Source: CAD feature listing. Evaluate the final solid. Frame: model axes, mm. A direction names the side the tool comes from. Give positions to 0.01 mm unless a question says otherwise; leave off trailing zeros. Loops run counter-clockwise (first coordinate to the right, second up) from the corner with the lowest first, then second, coordinate; pieces in that order, holes last. Notation, with made-up numbers: M 79.25,-28.75 L 101.25,-28.75 A21 ccw 101.25,10.25 Z; hole C 68.25,2.5 d7. An arc over 180 degrees is marked long. Write item = value, one per line.
from build123d import *

# Parameters (mm, degrees)
F0_W      = 315
F0_H      = 155
F1_DEPTH  = 105
F2_W      = 118
F2_H      = 80
F3_DEPTH  = 70
F4_W      = 65
F4_H      = 50
F5_DEPTH  = 57
F6_W      = 150
F6_H      = 15
F7_DEPTH  = 100
F8_W      = 150
F8_H      = 12
F9_DEPTH  = 75
F10_W     = 55
F10_H     = 28
F11_DEPTH = 55
F12_W     = 70
F12_H     = 30
F13_DEPTH = 100
F14_W     = 90
F14_H     = 20
F15_DEPTH = 90


with BuildPart() as f1:
    # F0 (on Top) → F1 (new body)
    with BuildSketch(Plane.XY):
        with Locations((-126.290321, 61.441531)):
            Rectangle(F0_W, F0_H)
    extrude(amount=F1_DEPTH)

    # F2 (on face) → F3 (cut)
    with BuildSketch(Plane.XY.offset(105)):
        with Locations((-41.790321, 37.941531)):
            Rectangle(F2_W, F2_H)
    extrude(amount=-F3_DEPTH, mode=Mode.SUBTRACT)

    # F4 (on face) → F5 (cut)
    with BuildSketch(Plane.XY.offset(105)):
        with Locations((-237.290321, 80.884401)):
            Rectangle(F4_W, F4_H)
    extrude(amount=-F5_DEPTH, mode=Mode.SUBTRACT)

    # F6 (on face) → F7 (cut)
    with BuildSketch(Plane.XY.offset(105)):
        with Locations((-194.790321, 5.441531)):
            Rectangle(F6_W, F6_H)
    extrude(amount=-F7_DEPTH, mode=Mode.SUBTRACT)

    # F8 (on face) → F9 (cut)
    with BuildSketch(Plane.XY.offset(105)):
        with Locations((-194.790321, 32.941531)):
            Rectangle(F8_W, F8_H)
    extrude(amount=-F9_DEPTH, mode=Mode.SUBTRACT)

    # F10 (on face) → F11 (cut)
    with BuildSketch(Plane.XY.offset(105)):
        with Locations((-147.290321, 66.941531)):
            Rectangle(F10_W, F10_H)
    extrude(amount=-F11_DEPTH, mode=Mode.SUBTRACT)

    # F12 (on face) → F13 (cut)
    with BuildSketch(Plane.XY.offset(105)):
        with Locations((-154.790321, 109.941531)):
            Rectangle(F12_W, F12_H)
    extrude(amount=-F13_DEPTH, mode=Mode.SUBTRACT)

    # F14 (on face) → F15 (cut)
    with BuildSketch(Plane.XY.offset(105)):
        with Locations((-55.790321, 104.941531)):
            Rectangle(F14_W, F14_H)
    extrude(amount=-F15_DEPTH, mode=Mode.SUBTRACT)


solid = f1.part
1. Cut plane C-C, the plane y = 99. Return the cut outline in (x, z).
Derived:
outline = M -283.79,0 L 31.21,0 L 31.21,105 L -10.79,105 L -10.79,15 L -100.79,15 L -100.79,105 L -119.79,105 L -119.79,5 L -189.79,5 L -189.79,105 L -204.79,105 L -204.79,48 L -269.79,48 L -269.79,105 L -283.79,105 Z
2. Cut plane A-A, the plane z = 22.5. Return the cut outline in (x, y), then the cut area to 3 significant figures.
Derived:
outline = M -283.79,-16.06 L 31.21,-16.06 L 31.21,138.94 L -283.79,138.94 Z; hole M -269.79,-2.06 L -119.79,-2.06 L -119.79,12.94 L -269.79,12.94 Z; hole M -189.79,94.94 L -119.79,94.94 L -119.79,124.94 L -189.79,124.94 Z; hole M -100.79,94.94 L -10.79,94.94 L -10.79,114.94 L -100.79,114.94 Z
area = 42,700 mm²
3. Material intervals for probe 1 along X at (y, z) = (35, 63.5); probe 2 along Y at (x, z) = (-44.5, 92); probe 3 along Y at (x, z) = (-202.5, 87), sorted ascending. Write a range as from..to.
Derived:
probe_1 = -283.79..-269.79, -119.79..-100.79, 17.21..31.21
probe_2 = -16.06..-2.06, 77.94..94.94, 114.94..138.94
probe_3 = -16.06..-2.06, 12.94..26.94, 38.94..138.94
4. Pull-direction query (Y, two-part tool) for faces 3 (the flat face through (-128, 138.942, 52)), 4 (the flat face through (-128, 45, 105)), 5 (the flat face through (-155, 110, 5)); classes: +Y half, -Y half, draft (parallel to the pull), parting line (faces both ways), or undercut.
Derived:
face_3 = +Y half
face_4 = draft
face_5 = undercut
5. Reachability of faces 1 (the flat face through (-196, 26.942, 68)), 2 (the flat face through (-283.79, 60, 52)) from +Z, -Z, +X, -X, +Y, -Y: full face, straight path, thin tool, end or side. Return the list, or none.
Derived:
face_1 = +Z
face_2 = +Z, -Z, -X, +Y, -Y
6. Cut plane D-D, the plane z = 68.5. Count the separate pieces of the cut face and the enclosed holes in it, then the cut area to 3 significant figures.
Derived:
separate_pieces = 1
enclosed_holes = 7
area = 26,600 mm²
7. Cut plane B-B, the plane x = -152. Return the cut outline in (y, z), then the cut area to 4 significant figures.
Derived:
outline = M -16.06,0 L 138.94,0 L 138.94,105 L 124.94,105 L 124.94,5 L 94.94,5 L 94.94,105 L 80.94,105 L 80.94,50 L 52.94,50 L 52.94,105 L 38.94,105 L 38.94,30 L 26.94,30 L 26.94,105 L 12.94,105 L 12.94,5 L -2.06,5 L -2.06,105 L -16.06,105 Z
area = 9,335 mm²
8. First-contact query: pin 1 Ø6 at (x, y) = (-213.5, 34) entering from +Z. Flat tip, straight axial feed; report the tip coordinate or a pass-through.
Derived:
pin_1 = 30
